```python
from build123d import *

# Parameters (mm, degrees)
F1_DEPTH      = 16
F4_ANGLE_BACK = 140
F4_ANGLE      = 280


with BuildPart() as f1:
    # F0 (on Top) → F1 (new body)
    with BuildSketch(Plane.XY):
        with BuildLine():
            Line((20.0751752723, -28.6703215501), (21.7959045813, -31.127777683))
            ThreePointArc((21.7959045813, -31.127777683), (32.9089653438, -19), (37.8553985275, -3.3119182244))
            ThreePointArc((37.8553985275, -3.3119182244), (32.9089653438, 19), (16.0594939461, 34.4396959074))
            ThreePointArc((16.0594939461, 34.4396959074), (0, 38), (-16.0594939461, 34.4396959074))
            ThreePointArc((-16.0594939461, 34.4396959074), (-32.9089653438, 19), (-37.8553985275, -3.3119182244))
            ThreePointArc((-37.8553985275, -3.3119182244), (-32.9089653438, -19), (-21.7959045813, -31.127777683))
            Line((-21.7959045813, -31.127777683), (-20.0751752723, -28.6703215501))
            ThreePointArc((-20.0751752723, -28.6703215501), (0, 35), (20.0751752723, -28.6703215501))
        make_face()
    extrude(amount=F1_DEPTH)

    # F3 (on Right) → F4 (revolve, cut)
    with BuildSketch(Plane.YZ, mode=Mode.PRIVATE) as f4_sk:
        Polygon((42.4908541927, 14.641066667), (38, 14.4704658035), (38, 13.5), (36.5, 12), (36.5, 4), (38, 2.5), (38, 0), (42.4908541927, 0), align=None)
    revolve(f4_sk.sketch.rotate(Axis((0, 0, 11.2814381719), (0, 0, -1)), -F4_ANGLE_BACK), axis=Axis((0, 0, 11.2814381719), (0, 0, -1)), revolution_arc=F4_ANGLE, mode=Mode.SUBTRACT)


solid = f1.part
```
Input: part model. Units: mm. Frame: model coordinates. A direction names the side the tool comes from. Coordinates: 2 decimals unless noted, no trailing zeros. Order: outer loops, then holes, each group sorted by start corner. A loop starts at its lowest first (then second) coordinate and runs counter-clockwise, first axis right, second up. Notation, with made-up numbers: (11, -3) - (51, -3) arc R19 ccw to (51, 3) - close; hole circle Ø7 at (81, 40.25). An arc over 180 degrees is marked (long way). Put each result on its own line as item: value.
1. Line query: line 1 along X through (y, z) = (0, 9.5); line 2 along Y through (x, z) = (0, 7.5); line 3 along X through (y, z) = (-10.5, 9). Output: solid intervals per line, ascending.
Report:
line 1: x = -36.5 to -35, 35 to 36.5
line 2: y = 35 to 36.5
line 3: x = -34.96 to -33.39, 33.39 to 34.96
2. Cut plane A-A on y = 0. Return the cut outline in (x, z).
Report:
outline: (-38, 0) - (-35, 0) - (-35, 16) - (-38, 16) - (-38, 13.5) - (-36.5, 12) - (-36.5, 4) - (-38, 2.5) - close; (35, 0) - (38, 0) - (38, 2.5) - (36.5, 4) - (36.5, 12) - (38, 13.5) - (38, 16) - (35, 16) - close
3. Draft query along Y for faces 1 (the face through (-9, 34, 16)), 2 (the face through (20.92, -29.88, 7.89)), 3 (the face through (-1.24, 34.98, 7.89)). Return one class per face: pulls with the +Y half, pulls with the -Y half, needs draft (parallel to the pull), parting line crosses it, or undercut.
Report:
face 1: needs draft
face 2: pulls with the -Y half
face 3: undercut
4. Contact query for flat-ended pins moving along their axis: pin 1 Ø5 at (y, z) = (8.5, 2) entering from +X; pin 2 Ø5 at (y, z) = (9, 4) entering from -X; pin 3 Ø5 at (x, z) = (-23, 4) entering from -Y. Output: stop coordinate, or through.
Report:
pin 1: stops at x = 37.52
pin 2: stops at x = -37.35
pin 3: stops at y = -31.13
5. Reachability of faces 4 (the face through (-20.95, -29.92, 7.89)), 5 (the face through (-1.26, 36.72, 12.24)), 6 (the face through (-9, 34, 0)) from +Z, -Z, +X, -X, +Y, -Y: full face, straight path, thin tool, end or side. Return the list, or none.
Report:
face 4: +Z, -Z, -Y
face 5: none
face 6: -Z, +X, -X, +Y, -Y
6. Cut plane C-C on z = 9. Return the cut outline in (x, y).
Report:
outline: (-24.43, -29.11) arc R38 ccw to (-21.8, -31.13) - (-20.08, -28.67) arc R35 cw (long way) to (20.08, -28.67) - (21.8, -31.13) arc R38 ccw to (24.43, -29.11) - (23.46, -27.96) arc R36.5 ccw (long way) to (-23.46, -27.96) - close
7. Cut plane B-B on x = 0. Return the cut outline in (y, z), then the cut area to 4 significant figures.
Report:
outline: (35, 0) - (38, 0) - (38, 2.5) - (36.5, 4) - (36.5, 12) - (38, 13.5) - (38, 16) - (35, 16) - close
area: 33.75 mm2
